Autodesk Inventor part; units mm, degrees
ref_plane "YZ Plane" through (0, 0, 0) normal (1, 0, 0) x (0, 1, 0)
ref_plane "XZ Plane" through (0, 0, 0) normal (0, 1, 0) x (-1, 0, 0)
ref_plane "XY Plane" through (0, 0, 0) normal (0, 0, 1) x (1, 0, 0)
sketch "Boceto1" plane through (0, 0, 0) normal (0, 0, 1) x (1, 0, 0)
  line L0 (0, 0) -> (10, 0)
  line L1 (10, 0) -> (10, -1.1604)
  line L2 (10, -1.1604) -> (12.5, -1.1604)
  line L3 (12.5, -1.1604) -> (12.5, -9.9104)
  line L4 (12.5, -9.9104) -> (33.5, -9.9104)
  line L5 (35.5, -7.9104) -> (35.5, 12.5896)
  line L6 (33.5, 14.5896) -> (12.5, 14.5896)
  line L7 (12.5, 14.5896) -> (12.5, 5.8396)
  line L8 (12.5, 5.8396) -> (10, 5.8396)
  line L9 (10, 5.8396) -> (10, 4)
  line L10 (10, 4) -> (0, 4)
  line L11 (0, 4) -> (0, 0)
  line L12 (37.5, 14.5896) -> (66.5, 14.5896)
  line L13 (66.5, 14.5896) -> (66.5, -9.9104)
  line L14 (66.5, -9.9104) -> (37.5, -9.9104)
  arc A0 (37.5, 14.5896) -> (35.5, 12.5896) centre (37.5, 12.5896) ccw
  arc A1 (35.5, -7.9104) -> (37.5, -9.9104) centre (37.5, -7.9104) ccw
  arc A2 (35.5, 12.5896) -> (33.5, 14.5896) centre (33.5, 12.5896) ccw
  arc A3 (33.5, -9.9104) -> (35.5, -7.9104) centre (33.5, -7.9104) ccw
  line L15 (66.5, 14.5896) -> (82, 14.5896)
  line L16 (84, 12.5896) -> (84, -7.9104)
  line L17 (82, -9.9104) -> (66.5, -9.9104)
  arc A4 (84, 12.5896) -> (82, 14.5896) centre (82, 12.5896) ccw
  arc A5 (82, -9.9104) -> (84, -7.9104) centre (82, -7.9104) ccw
  line L18 (-5.0848, 2) -> (93.2281, 2)
  point P0 (35.5, -9.9104)
  point P1 (35.5, 14.5896)
  point P2 (11.25, 5.8396)
  point P3 (11.25, -1.1604)
  point P4 (84, 14.5896)
  point P5 (0, 2)
  point P6 (84, 2)
  point P7 (35.5, 12.5896)
  dimension "d0" = 4
  dimension "d1" = 10
  dimension "d2" = 2.5
  dimension "d3" = 7
  dimension "d4" = 24.5
  dimension "d5" = 8.75
  dimension "d6" = 23
  dimension "d7" = 31
  dimension "d8" = 2
  dimension "d9" = 2
  dimension "d10" = 17.5
  dimension "d11" = 2
  dimension "d12" = 2
revolve "Revolución1" add sketch "Boceto1" angle 360 about axis through (-5.0848, 2, 0) along (1, 0, 0) contours L11 L10 L9 L8 L7 L6 A2 L5 L18 | L5 A0 L12 L13 L18 | L13 L15 A4 L16 L18
sketch "Boceto2" plane through (12.5, 2, 0) normal (-1, 0, 0) x (0, 0, 1)
  circle A0 centre (0, 8.5) radius 1.5
  circle A1 centre (0, -8.5) radius 1.5
  circle A2 centre (0, 0) radius 2
  point P0 (0, -2)
  dimension "d14" = 3
  dimension "d15" = 3
  dimension "d17" = 8.5
  dimension "d18" = 17
extrude "Extrusión1" cut sketch "Boceto2" against normal blind 15 contours A0 | A1
thread "Rosca1"
thread "Rosca2"
properties part number "Motor"
CAD build for the part. Positions are in the model's coordinates, mm. A direction names the side the tool comes from. Coordinates: 2 decimals unless noted, no trailing zeros. Loops run counter-clockwise (first coordinate to the right, second up) from the corner with the lowest first, then second, coordinate; pieces in that order, holes last. Notation, with made-up numbers: (-20.5, -13) - (33.5, -13) arc R14 cw to (33.5, 9) - close; hole circle Ø3 at (61.25, 24.5). An arc over 180 degrees is marked (long way). Use one line per item in the form item = value. Start each with the question number.
1) Tool access for faces 4 (the face through (11.232, 5.662, -1.153)), 5 (the face through (22.853, -10.577, -0.554)): list every direction of +Z, -Z, +X, -X, +Y, -Y with a clear straight run to the whole face (end or side of a thin tool).
2) Band-saw the part on C-C (y = 2). Give the cut face in (x, z), and give its area (3 significant figures).
3) Band-saw the part on D-D (x = 52). Give the cut face in (y, z), and give its area (3 significant figures).
4) Band-saw the part on B-B (x = 20). Give the cut face in (y, z), and give its area (3 significant figures).
5) Drill centre lines: L1, parallel to X at y = 8.75, z = 3.5; L2, parallel to X at y = 13.25, z = 0; L3, parallel to Y at x = 21.5, z = 4.5. Where is each one in solid material? Low to high. Write a range as from..to.
6) Flat gauge pins, fed straight in: pin 1 (5 mm diameter, centred on x = 68.5, z = -6.5, fed in from -Y); pin 2 (3.5 mm diameter, centred on y = -6.5, z = -0.5, fed in from -X); pin 3 (5 mm diameter, centred on x = 10.5, z = -8.5, fed in from +Y). Where does each tip first touch, or does it go through?
7) Band-saw the part on A-A (z = 0). Give the cut face in (x, y).
8) Two-plate mould, pull along Y, no slides. Class faces 1 (the face through (27.5, -6, 0)), 2 (the face through (10, 4, -2)), 3 (the face through (60.061, -10.577, 0.554)): +Y half, -Y half, draft (parallel to the pull), parting line (faces both ways), or undercut.
Check values:
q1.face_4 = -X
q1.face_5 = +X, -X
q2.outline = (0, -2) - (10, -2) - (10, -3.84) - (12.5, -3.84) - (12.5, -12.59) - (33.5, -12.59) arc R2 ccw to (35.5, -10.59) arc R2 ccw to (37.5, -12.59) - (82, -12.59) arc R2 ccw to (84, -10.59) - (84, 10.59) arc R2 ccw to (82, 12.59) - (37.5, 12.59) arc R2 ccw to (35.5, 10.59) arc R2 ccw to (33.5, 12.59) - (12.5, 12.59) - (12.5, 3.84) - (10, 3.84) - (10, 2) - (0, 2) - close
q2.area = 1,850 mm2
q3.outline = circle Ø25.18 at (2, 0)
q3.area = 498 mm2
q4.outline = circle Ø25.18 at (2, 0); hole circle Ø3 at (-6.5, 0); hole circle Ø3 at (10.5, 0)
q4.area = 484 mm2
q5.L1 = 12.5..84
q5.L2 = 12.5..35.39, 35.61..83.89
q5.L3 = -9.76..13.76
q6.pin_1 = -9.94
q6.pin_2 = 12.5
q6.pin_3 = 12.46
q7.outline = (0, 0) - (10, 0) - (10, -1.84) - (12.5, -1.84) - (12.5, -5) - (27.5, -5) - (27.5, -8) - (12.5, -8) - (12.5, -10.59) - (33.5, -10.59) arc R2 ccw to (35.5, -8.59) arc R2 ccw to (37.5, -10.59) - (82, -10.59) arc R2 ccw to (84, -8.59) - (84, 12.59) arc R2 ccw to (82, 14.59) - (37.5, 14.59) arc R2 ccw to (35.5, 12.59) arc R2 ccw to (33.5, 14.59) - (12.5, 14.59) - (12.5, 12) - (27.5, 12) - (27.5, 9) - (12.5, 9) - (12.5, 5.84) - (10, 5.84) - (10, 4) - (0, 4) - close
q8.face_1 = undercut
q8.face_2 = draft
q8.face_3 = parting line
